Read the model definition and answer for the solid it produces. Units are mm, in the model's axes. A direction names the side the tool comes from. Round coordinates to 2 decimals unless told otherwise and drop trailing zeros. Write each loop counter-clockwise with the first axis right and the second up, starting at its lowest first coordinate (ties: lowest second). Pieces come first, ordered by that corner, then holes. Notation, with made-up numbers: (-20, 45.5) - (-2, 45.5) arc R28 cw to (-2, 70.5) - close; hole circle Ø2 at (72.5, 1). An arc over 180 degrees is marked (long way). Answer as CSV lines item,"result". Start each with the question number.
1) For a pull along X with two mould halves and no side action, classify faces 3 (the cylindrical face through (23.179, 1.972, 37.116)), 4 (the cylindrical face through (0.217, 1.972, -12.244)), 5 (the flat face through (-1, 4, -8)) as +X half, -X half, draft (parallel to the pull), parting line (faces both ways), or undercut.
2) Find section C-C on y = 0.85. Determine the outline of the cut face in (x, z).
3) Which of the six approach directions +Z, -Z, +X, -X, +Y, -Y give full straight-line access (tool end or side, diameter ignored) to faces 1 (the flat face through (-4.893, 2, -32)), 2 (the flat face through (-1, 0, -8))?
4) Each of these flat-tipped pins is pushed along its axis until it touches: pin 1 (4 mm diameter, centred on x = 13, z = -47, fed in from -Y); pin 2 (1.2 mm diameter, centred on y = 1, z = -38, fed in from -X). Where does it stop, or does it pass through?
5) Find section D-D on x = 18. Determine the outline of the cut face in (y, z), then the cut area to 3 significant figures.
6) Find section A-A on z = -14. Determine the outline of the cut face in (x, y), then the cut area to 3 significant figures.
7) Find section B-B on x = 0.5. Determine the outline of the cut face in (y, z).
8) Consider line 1 along X through (y, z) = (0.75, -6); line 2 along X through (y, z) = (1.85, -41); line 3 along X through (y, z) = (0.45, -42.5). Determine where each line is inside the solid, lowest interval first.
from build123d import *

# Parameters (mm, degrees)
SKETCH1_R           = 50
BOSS_EXTRUDE1_DEPTH = 4


with BuildPart() as part:
    # Sketch1 → Boss-Extrude1 (new body)
    with BuildSketch(Plane(origin=(0, 0, 0), x_dir=(1, 0, 0), z_dir=(0, 1, 0))):
        with Locations((0.107420937, 7.243062526)):
            Circle(SKETCH1_R)
        with BuildLine():
            Line((-4.892579063, 17.243062526), (-4.892579063, 47.243062526))
            ThreePointArc((-4.892579063, 47.243062526), (0.107420937, 52.243062526), (5.107420937, 47.243062526))
            Line((5.107420937, 47.243062526), (5.107420937, 17.243062526))
            ThreePointArc((5.107420937, 17.243062526), (0.107420937, 12.243062526), (-4.892579063, 17.243062526))
        make_face(mode=Mode.SUBTRACT)
    extrude(amount=BOSS_EXTRUDE1_DEPTH)


solid = part.part
Check values:
1,face 3,"parting line"
1,face 4,"undercut"
1,face 5,"draft"
2,outline,"circle Ø100 at (0.11, -7.24); hole (-4.89, -47.24) arc R5 ccw to (5.11, -47.24) - (5.11, -17.24) arc R5 ccw to (-4.89, -17.24) - close"
3,face 1,"+Y, -Y"
3,face 2,"+Z, -Z, +X, -X, -Y"
4,pin 1,"stops at y = 0"
4,pin 2,"stops at x = -39.77"
5,outline,"(0, -53.93) - (4, -53.93) - (4, 39.45) - (0, 39.45) - close"
5,area,"374 mm^2"
6,outline,"(-49.43, 0) - (-3.7, 0) - (-3.7, 4) - (-49.43, 4) - close; (3.91, 0) - (49.65, 0) - (49.65, 4) - (3.91, 4) - close"
6,area,"366 mm^2"
7,outline,"(0, -57.24) - (4, -57.24) - (4, -52.23) - (0, -52.23) - close; (0, -12.26) - (4, -12.26) - (4, 42.76) - (0, 42.76) - close"
8,line 1,"x = -49.88 to 50.09"
8,line 2,"x = -36.78 to -4.89, 5.11 to 36.99"
8,line 3,"x = -35.35 to -4.89, 5.11 to 35.56"
